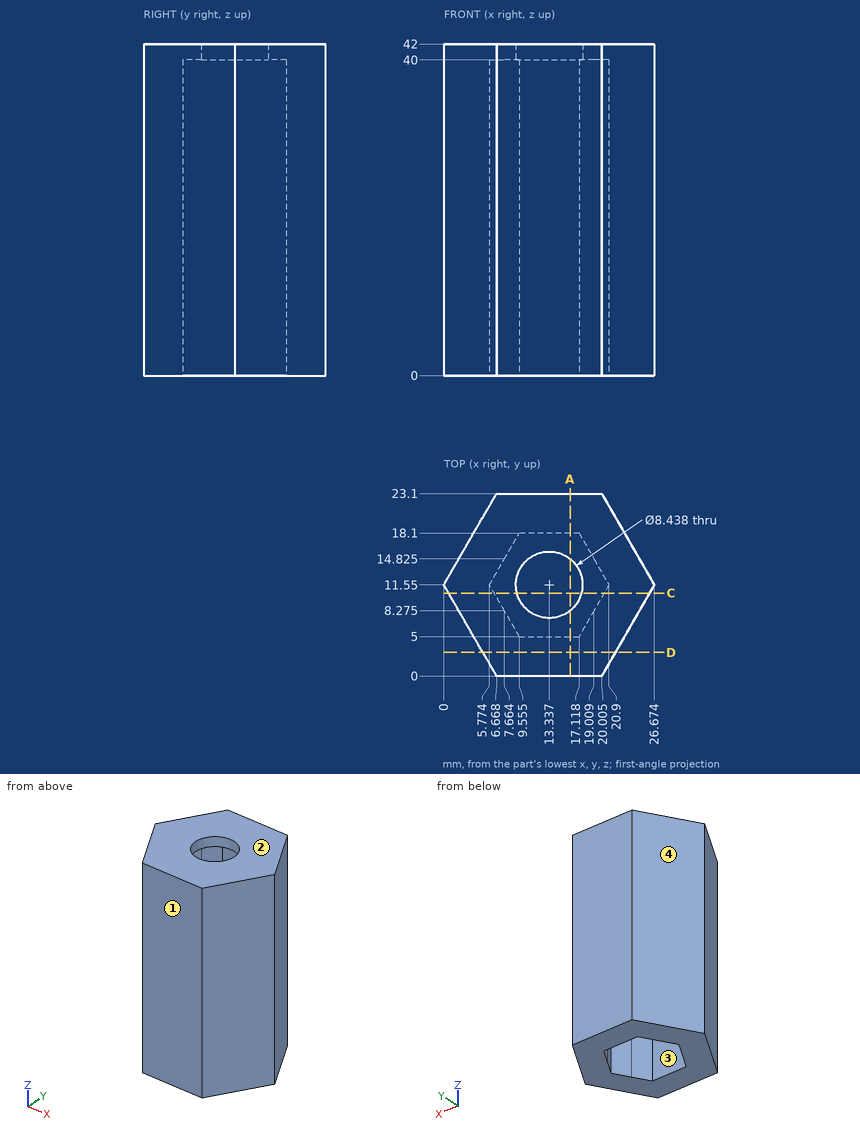
Drawing for the job (mm, zero at the part's lowest x, y, z). Give positions to 0.01 mm unless a question says otherwise; leave off trailing zeros. Write each loop counter-clockwise with the first axis right and the second up, starting at its lowest first coordinate (ties: lowest second). Pieces come first, ordered by that corner, then holes. Notation, with made-up numbers: M -36.5,35 L -31.5,35 A9 cw -31.5,50 Z; hole C -9,-20 d7. An arc over 180 degrees is marked long. Return JSON: item names as keys, results as strings. Group by question number.
(1) Band-saw the part on D-D (y = 3). Give the cut face in (x, z).
(2) Drill centre lines: L1, parallel to X at y = 11.55, z = 41.4 (1 decimal); L2, parallel to Y at x = 14.25, z = 28.5; L3, parallel to Y at x = 7, z = 8 (1 decimal). Where is each one in solid material? Low to high. Write a range as [from, to].
(3) Band-saw the part on C-C (y = 10.5). Give the cut face in (x, z).
(4) Flat gauge pins, fed straight in: pin 1 Ø2 at (y, z) = (9, 17.5) entering from +X; pin 2 Ø9.5 at (x, y) = (13.34, 11.55) entering from -Z; pin 3 Ø5 at (y, z) = (20.5, 18) entering from -X (1 decimal); pin 4 Ø2 at (x, y) = (14.5, 11) entering from +Z. Where does each tip first touch, or does it go through?
(5) Mould opens along Y. For the marked faces 1, 2, 3 and 4 say: pulls with the +Y half, pulls with the -Y half, needs draft (parallel to the pull), parting line crosses it, or undercut.
(6) Band-saw the part on A-A (x = 16). Give the cut face in (y, z).
Entries:
{
 "1": {"outline": "M 4.94,0 L 21.74,0 L 21.74,42 L 4.94,42 Z"},
 "2": {"L1": "x = [0, 9.1], [17.6, 26.7]", "L2": "y = [0, 5], [18.1, 23.1]", "L3": "y = [0, 9.4], [13.7, 23.1]"},
 "3": {"outline": "M 0.61,0 L 6.38,0 L 6.38,40 L 9.25,40 L 9.25,42 L 0.61,42 Z; M 17.42,40 L 20.29,40 L 20.29,0 L 26.07,0 L 26.07,42 L 17.42,42 Z"},
 "4": {"pin 1": "stops at x = 25.78", "pin 2": "stops at z = 40", "pin 3": "stops at x = 3.7", "pin 4": "passes through"},
 "5": {"face 1": "pulls with the -Y half", "face 2": "needs draft", "face 3": "undercut", "face 4": "pulls with the +Y half"},
 "6": {"outline": "M 0,0 L 5,0 L 5,40 L 8.28,40 L 8.28,42 L 0,42 Z; M 14.82,40 L 18.1,40 L 18.1,0 L 23.1,0 L 23.1,42 L 14.82,42 Z"}
}
